For this review, use the dimensioned drawing (mm, ordinates from the lowest corner) and the shaded views. Round coordinates to 2 decimals unless told otherwise and drop trailing zeros. Order: outer loops, then holes, each group sorted by start corner. A loop starts at its lowest first (then second) coordinate and runs counter-clockwise, first axis right, second up. Notation, with made-up numbers: (-3.75, -9) - (13.25, -9) arc R10 cw to (13.25, 10) - close; hole circle Ø1 at (84.25, -40). An arc over 180 degrees is marked (long way). Write item = value, one per line.
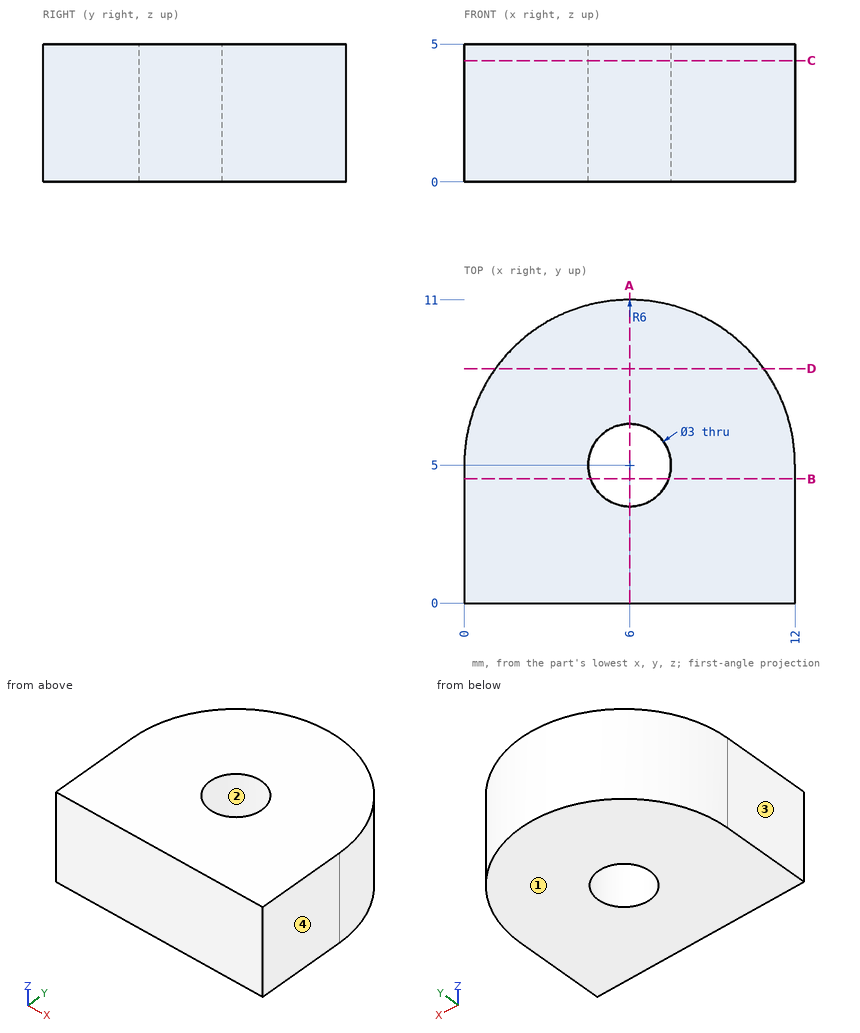
Item 1: Take a section at D-D, the plane y = 8.5. State the section outline as (x, z) points, and give its area (3 significant figures).
Data:
outline = (1.13, 0) - (10.87, 0) - (10.87, 5) - (1.13, 5) - close
area = 48.7 mm2
Item 2: Take a section at C-C, the plane z = 4.4. State the section outline as (x, y) points, and give its area (3 significant figures).
Data:
outline = (0, 0) - (12, 0) - (12, 5) arc R6 ccw to (0, 5) - close; hole circle Ø3 at (6, 5)
area = 109 mm2
Item 3: For line 1 along X through (y, z) = (5, 1.05); line 2 along Y through (x, z) = (6, 3.05); line 3 along X through (y, z) = (4, 3.3), list the stretches that pass through material, from the lowest coordinate up. Write a range as [from, to].
Data:
line_1 = [0, 4.5], [7.5, 12]
line_2 = [0, 3.5], [6.5, 11]
line_3 = [0, 4.88], [7.12, 12]
Item 4: The part is to be moulded in two halves that separate along X. For the marked faces 1, 2, 3 and 4, say which applies: +X half, -X half, draft (parallel to the pull), parting line (faces both ways), or undercut.
Data:
face_1 = draft
face_2 = undercut
face_3 = -X half
face_4 = +X half
Item 5: Take a section at A-A, the plane x = 6. State the section outline as (y, z) points, and give its area (3 significant figures).
Data:
outline = (0, 0) - (3.5, 0) - (3.5, 5) - (0, 5) - close; (6.5, 0) - (11, 0) - (11, 5) - (6.5, 5) - close
area = 40.0 mm2
Item 6: Take a section at B-B, the plane y = 4.5. State the section outline as (x, z) points.
Data:
outline = (0, 0) - (4.59, 0) - (4.59, 5) - (0, 5) - close; (7.41, 0) - (12, 0) - (12, 5) - (7.41, 5) - close
Item 7: Insertion check: P1, Ø2.5, axis at x = 6, y = 5, coming from the +Z side; P2, Ø1.5, axis at x = 2.5, z = 0.5, coming from the -Y side. Each pin has a flat end and moves straight along its axis. Give the tip position at first contact, or say it passes through.
Data:
P1 = through
P2 = 0
